Read the model definition and answer for the solid it produces. Units are mm, in the model's axes. A direction names the side the tool comes from. Coordinates: 2 decimals unless noted, no trailing zeros. Write each loop counter-clockwise with the first axis right and the second up, starting at its lowest first coordinate (ties: lowest second). Pieces come first, ordered by that corner, then holes. Notation, with made-up numbers: (-29.5, 45) -> (-8.5, 45) arc R26 ccw to (-8.5, 60) -> close; hole circle Ø2 at (36.25, 14.5). An arc over 180 degrees is marked (long way). Return JSON: item names as keys, results as strings.
from build123d import *

# Parameters (mm, degrees)
F2_DEPTH = 3.175
F3_DEPTH = 6.35


# Not quite as in the source:
# - a feature of the source that left no trace in its solid (it failed there, or was rolled back) is left out


with BuildPart() as f2:
    # F1 (on Front) → F2 (new body)
    with BuildSketch(Plane.XZ):
        with BuildLine():
            Line((38.1, 38.1), (-38.1, 38.1))
            ThreePointArc((-38.1, 38.1), (-42.5901280605, 36.2401280605), (-44.45, 31.75))
            Line((-44.45, 31.75), (-44.45, -44.45))
            ThreePointArc((-44.45, -44.45), (-42.5901280605, -48.9401280605), (-38.1, -50.8))
            Line((-38.1, -50.8), (38.1, -50.8))
            ThreePointArc((38.1, -50.8), (42.5901280605, -48.9401280605), (44.45, -44.45))
            Line((44.45, -44.45), (44.45, 31.75))
            ThreePointArc((44.45, 31.75), (42.5901280605, 36.2401280605), (38.1, 38.1))
        make_face()
    extrude(amount=F2_DEPTH)

    # F0 (on Front) → F3 (cut)
    with BuildSketch(Plane.XZ):
        with BuildLine():
            Line((-22.538606504, 15.2688146872), (23.1240657176, 15.1560609504))
            Line((23.1240657176, 15.1560609504), (23.1240657176, -29.7829657793))
            Line((23.1240657176, -29.7829657793), (13.8122134028, -29.7829657793))
            ThreePointArc((13.8122134028, -29.7829657793), (10.2694431158, -34.3118906021), (13.8122134028, -38.8408154249))
            Line((13.8122134028, -38.8408154249), (26.9613731652, -38.8408154249))
            ThreePointArc((26.9613731652, -38.8408154249), (30.4505025307, -36.6511380231), (31.8117402494, -32.7632410691))
            Line((31.8117402494, -32.7632410691), (31.8117402494, 17.4764426589))
            ThreePointArc((31.8117402494, 17.4764426589), (30.2845461796, 22.1904359309), (25.758318603, 24.2071952671))
            Line((25.758318603, 24.2071952671), (0, 24.2071952671))
            Line((0, 24.2071952671), (-25.758318603, 24.2071952671))
            ThreePointArc((-25.758318603, 24.2071952671), (-30.2845461796, 22.1904359309), (-31.8117402494, 17.4764426589))
            Line((-31.8117402494, 17.4764426589), (-31.8117402494, -32.7632410691))
            ThreePointArc((-31.8117402494, -32.7632410691), (-30.4505025307, -36.6511380231), (-26.9613731652, -38.8408154249))
            Line((-26.9613731652, -38.8408154249), (-0.5563573561, -38.8408154249))
            ThreePointArc((-0.5563573561, -38.8408154249), (2.7454534653, -37.1689483611), (4.597785615, -33.964894712))
            Line((4.597785615, -33.964894712), (4.597785615, -22.288704291))
            Line((4.597785615, -22.288704291), (12.7450192465, -16.3317304105))
            ThreePointArc((12.7450192465, -16.3317304105), (13.2165532375, -11.3368660938), (8.2683697798, -10.508316569))
            Line((8.2683697798, -10.508316569), (4.6611472023, -13.1736341055))
            Line((4.6611472023, -13.1736341055), (4.6611472023, -8.2560405135))
            ThreePointArc((4.6611472023, -8.2560405135), (0.8511472023, 6.6980150241), (-2.9588527977, -8.2560405135))
            Line((-2.9588527977, -8.2560405135), (-2.9588527977, -18.8035315381))
            Line((-2.9588527977, -18.8035315381), (-7.0704589598, -16.3561142981))
            ThreePointArc((-7.0704589598, -16.3561142981), (-11.4601778268, -17.9054311979), (-10.6000266969, -22.4803797901))
            Line((-10.6000266969, -22.4803797901), (-3.022214385, -27.0476285368))
            Line((-3.022214385, -27.0476285368), (-3.022214385, -29.7946484487))
            Line((-3.022214385, -29.7946484487), (-22.6497609527, -29.7461826206))
            Line((-22.6497609527, -29.7461826206), (-22.538606504, 15.2688146872))
        make_face()
    extrude(amount=F3_DEPTH, mode=Mode.SUBTRACT)


solid = f2.part
1. The part is cut by section A-A (x = 19.5). Determine the outline of the cut face in (y, z) (3 decimals), then the cut area to 3 significant figures.
Taken from the geometry:
{"outline": "(-3.175, -50.8) -> (0, -50.8) -> (0, -38.841) -> (-3.175, -38.841) -> close; (-3.175, -29.783) -> (0, -29.783) -> (0, 15.165) -> (-3.175, 15.165) -> close; (-3.175, 24.207) -> (0, 24.207) -> (0, 38.1) -> (-3.175, 38.1) -> close", "area": "225 mm2"}
2. The part is cut by section B-B (z = -35.5). Determine the outline of the cut face in (x, y) (3 decimals).
Taken from the geometry:
{"outline": "(-44.45, -3.175) -> (-31.179, -3.175) -> (-31.179, 0) -> (-44.45, 0) -> close; (4.017, -3.175) -> (10.423, -3.175) -> (10.423, 0) -> (4.017, 0) -> close; (31.179, -3.175) -> (44.45, -3.175) -> (44.45, 0) -> (31.179, 0) -> close"}
3. For a pull along Z with two mould halves and no side action, classify faces 1 (the face through (1.146, -1.565, 6.693)), 2 (the face through (-11, -3.175, -6)), 3 (the face through (42.64, -1.57, 36.19)) as +Z half, -Z half, draft (parallel to the pull), parting line (faces both ways), or undercut.
Taken from the geometry:
{"face 1": "undercut", "face 2": "draft", "face 3": "+Z half"}
4. The part is cut by section D-D (x = -29). Determine the outline of the cut face in (y, z) (3 decimals).
Taken from the geometry:
{"outline": "(-3.175, -50.8) -> (0, -50.8) -> (0, -37.973) -> (-3.175, -37.973) -> close; (-3.175, 23.272) -> (0, 23.272) -> (0, 38.1) -> (-3.175, 38.1) -> close"}
5. A flat-ended cylindrical pin translates along its axis: pin 1 Ø12.5 at (x, z) = (0.85, -1.26) entering from -Y. Find the tip coordinate at first contact, or state that the pin passes through.
Taken from the geometry:
{"pin 1": "passes through"}
6. A tool of negligible diameter and unlimited length cuts with its end or side. For faces 4 (the face through (44.45, -2, -7)), 5 (the face through (30.33, -1.57, 22.14)), from which of +Z, -Z, +X, -X, +Y, -Y can it reach the whole face along a straight path? Write none if from no direction.
Taken from the geometry:
{"face 4": "+Z, -Z, +X, +Y, -Y", "face 5": "+Y, -Y"}
7. Consider L1, parallel to Z at x = -17, y = -1.8; L2, parallel to X at y = -2.45, z = 11; L3, parallel to Z at x = -25, y = -0.4. Determine where each line is inside the solid, lowest interval first.
Taken from the geometry:
{"L1": "z = -50.8 to -38.84, -29.76 to 15.26, 24.21 to 38.1", "L2": "x = -44.45 to -31.81, -22.55 to 23.12, 31.81 to 44.45", "L3": "z = -50.8 to -38.84, 24.21 to 38.1"}
8. The part is cut by section C-C (z = 5.5). Determine the outline of the cut face in (x, y) (3 decimals), then the cut area to 3 significant figures.
Taken from the geometry:
{"outline": "(-44.45, -3.175) -> (-31.812, -3.175) -> (-31.812, 0) -> (-44.45, 0) -> close; (-22.563, -3.175) -> (-3.349, -3.175) -> (-3.349, 0) -> (-22.563, 0) -> close; (5.051, -3.175) -> (23.124, -3.175) -> (23.124, 0) -> (5.051, 0) -> close; (31.812, -3.175) -> (44.45, -3.175) -> (44.45, 0) -> (31.812, 0) -> close", "area": "199 mm2"}
